from build123d import *

# Parameters (mm, degrees)
SKETCH1_R           = 4
BOSS_EXTRUDE1_DEPTH = 3
SKETCH2_R           = 1.75
BOSS_EXTRUDE2_DEPTH = 15
FILLET2_R           = 1
SKETCH3_W           = 11.938810874
SKETCH3_H           = 2
CUT_EXTRUDE1_DEPTH  = 1
CHAMFER1_SIZE       = 1.75


with BuildPart() as part:
    # Sketch1 → Boss-Extrude1 (new body)
    with BuildSketch(Plane.XY):
        Circle(SKETCH1_R)
    extrude(amount=BOSS_EXTRUDE1_DEPTH)

    # Sketch2 → Boss-Extrude2 (add)
    with BuildSketch(Plane.XY.offset(3)):
        Circle(SKETCH2_R)
    extrude(amount=BOSS_EXTRUDE2_DEPTH)

    # Fillet2
    fillet2_edges = [part.edges().sort_by_distance(p)[0] for p in [
        (-4, 0, 0),
        (-4, 0, 3),
    ]]
    fillet(fillet2_edges, radius=FILLET2_R)

    # Sketch3 → Cut-Extrude1 (cut)
    with BuildSketch(Plane(origin=(0, 0, 0), x_dir=(-1, 0, 0), z_dir=(0, 0, -1))):
        with Locations((-0.202329925, 0)):
            Rectangle(SKETCH3_W, SKETCH3_H)
    extrude(amount=-CUT_EXTRUDE1_DEPTH, mode=Mode.SUBTRACT)

    # Chamfer1
    chamfer1_edges = [part.edges().sort_by_distance(p)[0] for p in [
        (-1.75, 0, 18),
    ]]
    chamfer(chamfer1_edges, length=CHAMFER1_SIZE)


solid = part.part
Check sheet for the modelled part. Datum: model origin and axes. Units: mm. A direction names the side the tool comes from. Give positions to 0.01 mm unless a question says otherwise; leave off trailing zeros. Loops run counter-clockwise (first coordinate to the right, second up) from the corner with the lowest first, then second, coordinate; pieces in that order, holes last. Notation, with made-up numbers: M 74,31.25 L 119,31.25 A22 ccw 119,70.25 Z; hole C 71.5,62 d7. An arc over 180 degrees is marked long. Return JSON: item names as keys, results as strings. Group by question number.
1. Mould release check, pull along Y, two halves, no side actions. Record for faces 4 (the flat face through (0.1, 1, 0.5)), 5 (the conical face through (0, 0, 18)), 6 (the flat face through (0, -2, 3)): released by +Y, released by -Y, zero draft, split by the parting line, or undercut.
2. Cross-section at A-A on z = 16. Record the boundary of the cut face in (x, y).
3. Tool access check on faces 1 (the flat face through (0.1, -1, 0.5)), 2 (the cylindrical face through (1.617, -0.67, 9.532)), 3 (the flat face through (0, -2, 0)). Record the directions out of +Z, -Z, +X, -X, +Y, -Y that give a thin tool (end or side, any length) a straight path to the whole face; none if there is none.
4. Go/stop test with flat-tipped pins: pin 1 (1.5 mm diameter, centred on x = -1.5, y = 0, fed in from -Z); pin 2 (1.5 mm diameter, centred on x = -1.5, z = 9.5, fed in from +Y); pin 3 (0.8 mm diameter, centred on x = -0.5, z = 0.5, fed in from +Y). Record where each tip stops, or that it passes through.
5. Cross-section at B-B on z = 1.5. Record the boundary of the cut face in (x, y), plus the area to 3 significant figures.
6. Thickness scan on L1, parallel to Z at x = -2, y = -2; L2, parallel to Z at x = -1.5, y = 0.25; L3, parallel to Y at x = -1.25, z = 5.75. Record the ranges inside material, lowest first.
Return value:
{
 "1": {"face 4": "undercut", "face 5": "split by the parting line", "face 6": "zero draft"},
 "2": {"outline": "C 0,0 d3.5"},
 "3": {"face 1": "-Z, +X, -X", "face 2": "+Z", "face 3": "-Z, +X, -X, +Y, -Y"},
 "4": {"pin 1": "z = 1", "pin 2": "y = 1.58", "pin 3": "y = 3.98"},
 "5": {"outline": "C 0,0 d8", "area": "50.3 mm^2"},
 "6": {"L1": "0 to 3", "L2": "1 to 16.48", "L3": "-1.22 to 1.22"}
}
